```python
from build123d import *

# Parameters (mm, degrees)
F0_W     = 101.6
F0_H     = 101.6
F1_DEPTH = 101.6
F2_W     = 12.7
F2_H     = 31.454976
F2_H_2   = 25.4
F2_W_2   = 25.4
F3_DEPTH = 101.6
F5_DEPTH = 101.6


with BuildPart() as f1:
    # F0 (on Top) → F1 (new body)
    with BuildSketch(Plane.XY):
        Rectangle(F0_W, F0_H)
    extrude(amount=F1_DEPTH)

    # F2 (on face) → F3 (cut)
    with BuildSketch(Plane(origin=(-50.8, 0, 0), x_dir=(0, -1, 0), z_dir=(-1, 0, 0))):
        with Locations((-44.45, 60.472512)):
            Rectangle(F2_W, F2_H)
        with Locations((44.45, 63.5)):
            Rectangle(F2_W, F2_H_2)
        with Locations((-12.7, 12.7)):
            Rectangle(F2_W_2, F2_H_2)
        with Locations((12.7, 12.7)):
            Rectangle(F2_W_2, F2_H_2)
    extrude(amount=-F3_DEPTH, mode=Mode.SUBTRACT)

    # F4 (on face) → F5 (cut)
    with BuildSketch(Plane(origin=(-50.8, 0, 0), x_dir=(0, -1, 0), z_dir=(-1, 0, 0))):
        Polygon((0, 101.6), (-25.4, 101.6), (0, 76.2), align=None)
        Polygon((25.4, 101.6), (0, 101.6), (0, 76.2), align=None)
    extrude(amount=-F5_DEPTH, mode=Mode.SUBTRACT)


solid = f1.part
```
Source: CAD feature listing. Evaluate the final solid. Frame: model axes, mm. A direction names the side the tool comes from. Coordinates: 2 decimals unless noted, no trailing zeros. Loops run counter-clockwise (first coordinate to the right, second up) from the corner with the lowest first, then second, coordinate; pieces in that order, holes last. Notation, with made-up numbers: M -3,81.5 L 42,81.5 A9 ccw 42,88.5 Z; hole C 37.5,42.25 d6. An arc over 180 degrees is marked long. Use CSV: the item, a comma, the result in double quotes.
(1) Cut plane D-D on y = 10.5. Return loops of the section in (x, z).
Answers follow:
outline,"M -50.8,25.4 L 50.8,25.4 L 50.8,86.7 L -50.8,86.7 Z"
(2) Cut plane C-C on z = 83.5. Return loops of the section in (x, y), and give its area (3 significant figures).
Answers follow:
outline,"M -50.8,-50.8 L 50.8,-50.8 L 50.8,-7.3 L -50.8,-7.3 Z; M -50.8,7.3 L 50.8,7.3 L 50.8,50.8 L -50.8,50.8 Z"
area,"8,840 mm²"
(3) Line query: line 1 (Y direction, x = 24, z = 24); line 2 (Z direction, x = -12.5, y = -45.5); line 3 (Z direction, x = -37, y = 0). Output: solid intervals per line, ascending. Write a range as [from, to].
Answers follow:
line 1,"[-50.8, -25.4], [25.4, 50.8]"
line 2,"[0, 50.8], [76.2, 101.6]"
line 3,"[25.4, 76.2]"
(4) Contact query for flat-ended pins moving along their axis: pin 1 (25 mm diameter, centred on x = 25, z = 60.5, fed in from +Y); pin 2 (3 mm diameter, centred on y = -40, z = 70.5, fed in from +X); pin 3 (7.5 mm diameter, centred on x = 20.5, z = 57.5, fed in from -Y); pin 4 (1 mm diameter, centred on x = -39.5, y = -17, fed in from +Z). Output: stop coordinate, or through.
Answers follow:
pin 1,"y = 38.1"
pin 2,"through"
pin 3,"y = -38.1"
pin 4,"z = 93.7"
(5) Reachability of faces 1 (the face through (-0.7, -12.5, 88.7)), 2 (the face through (-1, 38.1, 60)), 3 (the face through (-1, -44, 76.2)) from +Z, -Z, +X, -X, +Y, -Y: full face, straight path, thin tool, end or side. Return the list, or none.
Answers follow:
face 1,"+Z, +X, -X"
face 2,"+X, -X, +Y"
face 3,"+X, -X, -Y"
(6) Cut plane A-A on z = 12.5. Return loops of the section in (x, y).
Answers follow:
outline,"M -50.8,-50.8 L 50.8,-50.8 L 50.8,-25.4 L -50.8,-25.4 Z; M -50.8,25.4 L 50.8,25.4 L 50.8,50.8 L -50.8,50.8 Z"
(7) Cut plane B-B on x = 29. Return loops of the section in (y, z), and give its area (4 significant figures).
Answers follow:
outline,"M -50.8,0 L -25.4,0 L -25.4,25.4 L 25.4,25.4 L 25.4,0 L 50.8,0 L 50.8,44.75 L 38.1,44.75 L 38.1,76.2 L 50.8,76.2 L 50.8,101.6 L 25.4,101.6 L 0,76.2 L -25.4,101.6 L -50.8,101.6 L -50.8,76.2 L -38.1,76.2 L -38.1,50.8 L -50.8,50.8 Z"
area,"7,665 mm²"
(8) Draft query along Z for faces 4 (the face through (-1, -44, 50.8)), 5 (the face through (-1, -38, 101.6)), 6 (the face through (-1, -25.4, 13)), 7 (the face through (-1, 45, 44.745)). Return one class per face: pulls with the +Z half, pulls with the -Z half, needs draft (parallel to the pull), parting line crosses it, or undercut.
Answers follow:
face 4,"undercut"
face 5,"pulls with the +Z half"
face 6,"needs draft"
face 7,"undercut"
